```python
from build123d import *

# Parameters (mm, degrees)
FRAME_SKETCH_R           = 1.5
FRAME_SKETCH_R_2         = 1
FRAME_BOTTOM_PLATE_DEPTH = 4


with BuildPart() as part:
    # Frame Sketch → Frame Bottom Plate (new body)
    with BuildSketch(Plane(origin=(0, 0, 0), x_dir=(1, 0, 0), z_dir=(0, 1, 0))):
        with BuildLine():
            Line((18.280787571, 56.140393786), (-13.719212429, 56.140393786))
            ThreePointArc((-13.719212429, 56.140393786), (-14.42631921, 55.847500567), (-14.719212429, 55.140393786))
            Line((-14.719212429, 55.140393786), (-14.719212429, 49.140393786))
            Line((-14.719212429, 49.140393786), (-49.176727046, 102.27090579))
            Line((-49.176727046, 102.27090579), (-49.176727046, 81.27090579))
            Line((-49.176727046, 81.27090579), (-14.719212429, 26.140393786))
            Line((-14.719212429, 26.140393786), (-14.719212429, 0.140393786))
            Line((-14.719212429, 0.140393786), (-49.176727046, -54.990118218))
            Line((-49.176727046, -54.990118218), (-49.176727046, -75.990118218))
            Line((-49.176727046, -75.990118218), (-14.719212429, -22.859606214))
            Line((-14.719212429, -22.859606214), (-14.719212429, -54.859606214))
            ThreePointArc((-14.719212429, -54.859606214), (-14.42631921, -55.566712995), (-13.719212429, -55.859606214))
            Line((-13.719212429, -55.859606214), (18.280787571, -55.859606214))
            ThreePointArc((18.280787571, -55.859606214), (18.987894353, -55.566712995), (19.280787571, -54.859606214))
            Line((19.280787571, -54.859606214), (19.280787571, -22.859606214))
            Line((19.280787571, -22.859606214), (53.738302189, -75.990118218))
            Line((53.738302189, -75.990118218), (53.738302189, -54.990118218))
            Line((53.738302189, -54.990118218), (19.280787571, 0.140393786))
            Line((19.280787571, 0.140393786), (19.280787571, 26.140393786))
            Line((19.280787571, 26.140393786), (53.738302189, 81.27090579))
            Line((53.738302189, 81.27090579), (53.738302189, 102.27090579))
            Line((53.738302189, 102.27090579), (19.280787571, 49.140393786))
            Line((19.280787571, 49.140393786), (19.280787571, 55.140393786))
            ThreePointArc((19.280787571, 55.140393786), (18.987894353, 55.847500567), (18.280787571, 56.140393786))
        make_face()
        with Locations(Location((-12.219212429, -52.959606214, 0), (0, 0, 270))):
            Circle(FRAME_SKETCH_R, mode=Mode.SUBTRACT)
        with BuildLine():
            Line((9.421181357, -46.859606214), (-4.859606214, -46.859606214))
            ThreePointArc((-4.859606214, -46.859606214), (-5.467439598, -46.607833383), (-5.719212429, -46))
            Line((-5.719212429, -46), (-5.719212429, -34.359606214))
            ThreePointArc((-5.719212429, -34.359606214), (-4.986979382, -32.591839261), (-3.219212429, -31.859606214))
            Line((-3.219212429, -31.859606214), (7.780787571, -31.859606214))
            ThreePointArc((7.780787571, -31.859606214), (9.548554524, -32.591839261), (10.280787571, -34.359606214))
            Line((10.280787571, -34.359606214), (10.280787571, -46))
            ThreePointArc((10.280787571, -46), (10.02901474, -46.607833383), (9.421181357, -46.859606214))
        make_face(mode=Mode.SUBTRACT)
        with Locations(Location((16.780787571, -52.959606214, 0), (0, 0, 270))):
            Circle(FRAME_SKETCH_R, mode=Mode.SUBTRACT)
        with BuildLine():
            ThreePointArc((10.780787571, -23.859606214), (10.195001134, -25.273819777), (8.780787571, -25.859606214))
            Line((8.780787571, -25.859606214), (-4.219212429, -25.859606214))
            ThreePointArc((-4.219212429, -25.859606214), (-5.633425991, -25.273819777), (-6.219212429, -23.859606214))
            Line((-6.219212429, -23.859606214), (-6.219212429, -12.359606214))
            ThreePointArc((-6.219212429, -12.359606214), (-5.194086163, -9.88473248), (-2.719212429, -8.859606214))
            Line((-2.719212429, -8.859606214), (7.280787571, -8.859606214))
            ThreePointArc((7.280787571, -8.859606214), (9.755661306, -9.88473248), (10.780787571, -12.359606214))
            Line((10.780787571, -12.359606214), (10.780787571, -23.859606214))
        make_face(mode=Mode.SUBTRACT)
        with BuildLine():
            Line((6.780787571, 8.140393786), (-2.219212429, 8.140393786))
            ThreePointArc((-2.219212429, 8.140393786), (-4.694086163, 9.165520052), (-5.719212429, 11.640393786))
            Line((-5.719212429, 11.640393786), (-5.719212429, 21.640393786))
            ThreePointArc((-5.719212429, 21.640393786), (-4.694086163, 24.11526752), (-2.219212429, 25.140393786))
            Line((-2.219212429, 25.140393786), (6.780787571, 25.140393786))
            ThreePointArc((6.780787571, 25.140393786), (9.255661306, 24.11526752), (10.280787571, 21.640393786))
            Line((10.280787571, 21.640393786), (10.280787571, 11.640393786))
            ThreePointArc((10.280787571, 11.640393786), (9.255661306, 9.165520052), (6.780787571, 8.140393786))
        make_face(mode=Mode.SUBTRACT)
        with Locations(Location((-8.469212429, 46.240393786, 0), (0, 0, 270))):
            Circle(FRAME_SKETCH_R_2, mode=Mode.SUBTRACT)
        with BuildLine():
            Line((5.530787571, 35.140393786), (-0.969212429, 35.140393786))
            ThreePointArc((-0.969212429, 35.140393786), (-2.736979382, 35.872626833), (-3.469212429, 37.640393786))
            Line((-3.469212429, 37.640393786), (-3.469212429, 49.140393786))
            ThreePointArc((-3.469212429, 49.140393786), (-3.17631921, 49.847500567), (-2.469212429, 50.140393786))
            Line((-2.469212429, 50.140393786), (7.030787571, 50.140393786))
            ThreePointArc((7.030787571, 50.140393786), (7.737894353, 49.847500567), (8.030787571, 49.140393786))
            Line((8.030787571, 49.140393786), (8.030787571, 37.640393786))
            ThreePointArc((8.030787571, 37.640393786), (7.298554524, 35.872626833), (5.530787571, 35.140393786))
        make_face(mode=Mode.SUBTRACT)
        with Locations(Location((-8.469212429, 51.140393786, 0), (0, 0, 270))):
            Circle(FRAME_SKETCH_R_2, mode=Mode.SUBTRACT)
        with Locations(Location((13.030787571, 46.240393786, 0), (0, 0, 270))):
            Circle(FRAME_SKETCH_R_2, mode=Mode.SUBTRACT)
        with Locations(Location((13.030787571, 51.140393786, 0), (0, 0, 270))):
            Circle(FRAME_SKETCH_R_2, mode=Mode.SUBTRACT)
    extrude(amount=FRAME_BOTTOM_PLATE_DEPTH)


solid = part.part
```
Design review of the part built by this model. Coordinates are the model's own, in mm. A direction names the side the tool comes from. Round coordinates to 2 decimals unless told otherwise and drop trailing zeros. Order: outer loops, then holes, each group sorted by start corner. A loop starts at its lowest first (then second) coordinate and runs counter-clockwise, first axis right, second up. Notation, with made-up numbers: (-13, 45) - (5, 45) arc R22 ccw to (5, 57) - close; hole circle Ø7 at (84, 23.5). An arc over 180 degrees is marked (long way). Return JSON: item names as keys, results as strings.
Q1. Machinability: for faces 5 (the flat face through (2, 2, 8.86)), 6 (the flat face through (36.75, 1.97, 27.81)), 7 (the flat face through (36.75, 1.97, -76.08)), 8 (the flat face through (-32.19, 1.97, -54.09)), 9 (the flat face through (-32.19, 1.97, 49.8)), which of the approach directions +Z, -Z, +X, -X, +Y, -Y give a long, thin tool a straight path to every point of the face, cutting with its end or side? Answer none if there is none.
Computed values:
{"face 5": "+Y, -Y", "face 6": "+X, +Y, -Y", "face 7": "-Z, +Y, -Y", "face 8": "-X, +Y, -Y", "face 9": "+Z, +Y, -Y"}
Q2. For pin 1 Ø2 at (x, y) = (4.5, 1) entering from +Z; pin 2 Ø2 at (y, z) = (2, 19.5) entering from -X; pin 3 Ø1.2 at (y, z) = (3, 39) entering from +X; pin 4 Ø1 at (x, z) = (-11.5, -53.5) entering from -Y, all flat-tipped, find the tip position at first contact; note any pin that passes through.
Computed values:
{"pin 1": "stops at z = 55.86", "pin 2": "stops at x = -27.62", "pin 3": "stops at x = 44.12", "pin 4": "stops at y = 0"}
Q3. Consider section A-A on z = -84.5. Write out the cut boundary in (x, y), plus the area to 3 significant figures.
Computed values:
{"outline": "(-49.18, 0) - (-37.65, 0) - (-37.65, 4) - (-49.18, 4) - close; (42.21, 0) - (53.74, 0) - (53.74, 4) - (42.21, 4) - close", "area": "92.2 mm2"}
Q4. Wall thickness on L1, parallel to X at y = 1.45, z = -51; L2, parallel to X at y = 2.35, z = 28.5; L3, parallel to X at y = 1.35, z = -46: over which ranges is each line inside the solid? List them lowest first. Write a range as [from, to].
Computed values:
{"L1": "x = [-30.26, -15.93], [-14.72, -9.46], [-7.48, 12.04], [14.02, 19.28], [20.49, 34.82]", "L2": "x = [-32.62, -18.38], [-14.72, 19.28], [22.94, 37.18]", "L3": "x = [-27.13, -9.44], [-7.5, -3.47], [8.03, 12.06], [14, 31.69]"}
Q5. Consider section C-C on y = 3.25. Give the number of separate pieces and of enclosed holes in the cut face, plus the area to 3 significant figures.
Computed values:
{"separate pieces": "1", "enclosed holes": "10", "area": "5,860 mm2"}
Q6. Consider section B-B on x = -22. Write out the cut boundary in (y, z), plus the area to 3 significant figures.
Computed values:
{"outline": "(0, -60.37) - (4, -60.37) - (4, -37.79) - (0, -37.79) - close; (0, 11.51) - (4, 11.51) - (4, 34.09) - (0, 34.09) - close", "area": "181 mm2"}
Q7. The part is to be moulded in two halves that separate along X. For faces 1 (the flat face through (-49.177, 2, -92)), 2 (the flat face through (13, 0, -14)), 3 (the flat face through (-6.219, 2, 18)), 4 (the flat face through (-14.719, 2, 39)), say which applies: pulls with the +X half, pulls with the -X half, needs draft (parallel to the pull), parting line crosses it, or undercut.
Computed values:
{"face 1": "pulls with the -X half", "face 2": "needs draft", "face 3": "undercut", "face 4": "undercut"}
